Check sheet for the modelled part. Datum: model origin and axes. Units: mm. Coordinates: 2 decimals unless noted, no trailing zeros. Write each loop counter-clockwise with the first axis right and the second up, starting at its lowest first coordinate (ties: lowest second). Pieces come first, ordered by that corner, then holes. Notation, with made-up numbers: (-20, 10) - (36, 10) arc R16 ccw to (36, 20) - close; hole circle Ø7 at (47, 88). An arc over 180 degrees is marked (long way). Answer as CSV lines item,"result". Start each with the question number.
from build123d import *

# Parameters (mm, degrees)
SKETCH1_R           = 59.99988
SKETCH1_R_2         = 17.145
SKETCH1_R_3         = 3.175
BOSS_EXTRUDE1_DEPTH = 5
SKETCH2_R           = 5.59943
CUT_EXTRUDE1_DEPTH  = 6
CIRPATTERN1_COUNT   = 6


with BuildPart() as part:
    # Sketch1 → Boss-Extrude1 (new body)
    with BuildSketch(Plane(origin=(0, 0, 0), x_dir=(1, 0, 0), z_dir=(0, 1, 0))):
        Circle(SKETCH1_R)
        Circle(SKETCH1_R_2, mode=Mode.SUBTRACT)
        with Locations((21.997045256, -12.7)):
            Circle(SKETCH1_R_3, mode=Mode.SUBTRACT)
        with Locations((0, 25.4)):
            Circle(SKETCH1_R_3, mode=Mode.SUBTRACT)
        with Locations((-21.997045256, -12.7)):
            Circle(SKETCH1_R_3, mode=Mode.SUBTRACT)
    extrude(amount=BOSS_EXTRUDE1_DEPTH)

    # Sketch2 → Cut-Extrude1 (cut, through all)
    with BuildSketch(Plane(origin=(0, 5, 0), x_dir=(1, 0, 0), z_dir=(0, 1, 0))):
        with Locations((0, 59.99988)):
            Circle(SKETCH2_R)
    cut_extrude1 = extrude(amount=-CUT_EXTRUDE1_DEPTH, mode=Mode.SUBTRACT)

    # CirPattern1: Cut-Extrude1 ×6 about axis
    cirpattern1_axis = Axis((0, 0, 0), (0, 1, 0))
    for i in range(1, CIRPATTERN1_COUNT):
        add(cut_extrude1.rotate(cirpattern1_axis, i * 360 / CIRPATTERN1_COUNT), mode=Mode.SUBTRACT)


solid = part.part
(1) Cross-section at D-D on z = 12.7. Record the boundary of the cut face in (x, y).
(2) Release check for a two-part mould opening along X. For faces 1 (the face through (-19.064, 2.465, 13.916)), 2 (the face through (-30.31, 2.46, 51.78)), 3 (the face through (29.69, 2.46, 52.14)) record: pulls with the +X half, pulls with the -X half, needs draft (parallel to the pull), parting line crosses it, or undercut.
(3) Material ranges on probe 1 along Z at (x, y) = (0, 2.35) (3 decimals); probe 2 along X at (y, z) = (3.2, 0) (3 decimals); probe 3 along Z at (x, y) = (-2.5, 1.85), recorded low to high. Write a range as from..to.
(4) Go/stop test with flat-tipped pins: P1, Ø5.5, axis at x = 22, z = 12.7, coming from the -Y side; P2, Ø1.5, axis at y = 2.5, z = 42, coming from the -X side; P3, Ø2, axis at x = 44, y = 2.5, coming from the +Z side. Record where each tip stops, or that it passes through.
(5) Cross-section at B-B on y = 4.2. Record the boundary of the cut face in (x, z) (3 decimals).
(6) Cross-section at C-C on z = 0. Record the boundary of the cut face in (x, y) (3 decimals).
(7) Cross-section at A-A on x = 0. Record the boundary of the cut face in (y, z) (3 decimals).
Checked values:
1,outline,"(-58.64, 0) - (-25.17, 0) - (-25.17, 5) - (-58.64, 5) - close; (-18.82, 0) - (-11.52, 0) - (-11.52, 5) - (-18.82, 5) - close; (11.52, 0) - (18.82, 0) - (18.82, 5) - (11.52, 5) - close; (25.17, 0) - (58.64, 0) - (58.64, 5) - (25.17, 5) - close"
2,face 1,"undercut"
2,face 2,"pulls with the -X half"
2,face 3,"pulls with the +X half"
3,probe 1,"-54.4..-28.575, -22.225..-17.145, 17.145..54.4"
3,probe 2,"-60..-17.145, 17.145..60"
3,probe 3,"-54.99..-27.36, -23.44..-16.96, 16.96..54.99"
4,P1,"through"
4,P2,"x = -43.57"
4,P3,"z = 41.84"
5,outline,"(-54.532, -25.025) arc R5.599 cw to (-48.938, -34.713) arc R60 ccw to (-5.593, -59.739) arc R5.599 cw to (5.593, -59.739) arc R60 ccw to (48.938, -34.713) arc R5.599 cw to (54.532, -25.025) arc R60 ccw to (54.532, 25.025) arc R5.599 cw to (48.938, 34.713) arc R60 ccw to (5.593, 59.739) arc R5.599 cw to (-5.593, 59.739) arc R60 ccw to (-48.938, 34.713) arc R5.599 cw to (-54.532, 25.025) arc R60 ccw to start; hole circle Ø6.35 at (-21.997, 12.7); hole circle Ø34.29 at (0, 0); hole circle Ø6.35 at (0, -25.4); hole circle Ø6.35 at (21.997, 12.7)"
6,outline,"(-60, 0) - (-17.145, 0) - (-17.145, 5) - (-60, 5) - close; (17.145, 0) - (60, 0) - (60, 5) - (17.145, 5) - close"
7,outline,"(0, -54.4) - (5, -54.4) - (5, -28.575) - (0, -28.575) - close; (0, -22.225) - (5, -22.225) - (5, -17.145) - (0, -17.145) - close; (0, 17.145) - (5, 17.145) - (5, 54.4) - (0, 54.4) - close"
